Autodesk Inventor part; units mm, degrees
ref_plane "YZ Plane" through (0, 0, 0) normal (1, 0, 0) x (0, 1, 0)
ref_plane "XZ Plane" through (0, 0, 0) normal (0, 1, 0) x (-1, 0, 0)
ref_plane "XY Plane" through (0, 0, 0) normal (0, 0, 1) x (1, 0, 0)
sketch "Sketch1" plane through (0, 0, 0) normal (1, 0, 0) x (0, 1, 0)
  line L0 (-11.2229, 4.9257) -> (471.3771, 4.9257)
  line L1 (471.3771, 4.9257) -> (471.3771, -7.7743)
  line L2 (471.3771, -7.7743) -> (-11.2229, -7.7743)
  line L3 (-11.2229, -7.7743) -> (-11.2229, 4.9257)
  point P0 (0, 0)
  dimension "d0" = 482.6
revolve "Revolution1" add sketch "Sketch1" angle 360 about axis through (0, -11.2229, 4.9257) along (0, 1, 0)
sketch "Sketch2" plane through (0, 471.3771, 4.9257) normal (0, 1, 0) x (1, 0, 0)
  line L0 (-2.5588, -10.1161) -> (2.6183, -10.1161)
  line L1 (2.6183, -10.1161) -> (2.6183, 10.1161)
  line L2 (2.6183, 10.1161) -> (-2.5588, 10.1161)
  line L3 (-2.5588, 10.1161) -> (-2.5588, -10.1161)
  line L4 (-2.5588, 0) -> (2.6183, 0)
  point P0 (0, 4.9257)
extrude "Extrusion1" add sketch "Sketch2" along normal blind 95.25
sketch "Sketch3" plane through (2.6183, 471.3771, 15.0418) normal (1, 0, 0) x (0, 0, -1)
  line L0 (20.2322, 0) -> (0, 0)
  line L1 (20.2322, 0) -> (20.2322, 95.25)
  line L2 (0, 95.25) -> (20.2322, 95.25)
  line L3 (0, 0) -> (0, 95.25)
  line L4 (-2.5839, 0) -> (22.8161, 0)
  line L5 (10.1161, 0) -> (10.1161, 76.2)
  circle A0 centre (10.1161, 76.2) radius 12.7
  circle A1 centre (10.1161, 76.2) radius 19.05
  point P0 (15.0418, -471.3771)
  dimension "d10" = 76.2
  dimension "d11" = 25.4
  dimension "d12" = 38.1
extrude "Extrusion2" add sketch "Sketch3" against normal blind 6.35 contours A1 L5 A0 L1 | L1 A0 A1 | A1 L3 A0 L5 | A1 L3 A0 | A0 L3 A1 L1
sketch "Sketch4" plane through (2.6183, 471.3771, 15.0418) normal (1, 0, 0) x (0, 0, -1)
  line L0 (20.2322, 68.5218) -> (20.2322, 83.8782)
  arc A0 (20.2322, 68.5218) -> (20.2322, 83.8782) centre (10.1161, 76.2) ccw
  arc A1 (20.2322, 60.0579) -> (20.2322, 92.3421) centre (10.1161, 76.2) ccw
  line L1 (20.2322, 92.3421) -> (20.2322, 95.25)
  line L2 (0, 95.25) -> (20.2322, 95.25)
  line L3 (0, 92.3421) -> (0, 95.25)
  arc A2 (0, 92.3421) -> (0, 60.0579) centre (10.1161, 76.2) ccw
  line L4 (0, 0) -> (0, 60.0579)
  line L5 (20.2322, 0) -> (0, 0)
  line L6 (20.2322, 0) -> (20.2322, 60.0579)
  arc A3 (0, 83.8782) -> (0, 68.5218) centre (10.1161, 76.2) ccw
  line L7 (0, 68.5218) -> (0, 83.8782)
  arc A4 (0, 83.8782) -> (0, 68.5218) centre (10.1161, 76.2) ccw
  arc A5 (20.2322, 83.8782) -> (0, 83.8782) centre (10.1161, 76.2) ccw
  arc A6 (20.2322, 68.5218) -> (20.2322, 83.8782) centre (10.1161, 76.2) ccw
  arc A7 (0, 68.5218) -> (20.2322, 68.5218) centre (10.1161, 76.2) ccw
  circle A8 centre (10.1161, 76.2) radius 12.7
  point P0 (15.0418, -471.3771)
extrude "Extrusion3" cut sketch "Sketch4" against normal blind 6.35 contours A7 L7 A5 L0 | L0 A0 | A3 L7
properties part number "Rod"
For this review, take the finished solid that the model builds, in its own axes (mm). A direction names the side the tool comes from. Round coordinates to 2 decimals unless told otherwise and drop trailing zeros. Order: outer loops, then holes, each group sorted by start corner. A loop starts at its lowest first (then second) coordinate and runs counter-clockwise, first axis right, second up. Notation, with made-up numbers: M 55,-28.5 L 73,-28.5 A19 ccw 73,-16.5 Z; hole C -25.75,82.5 d10. An arc over 180 degrees is marked long. Use a Markdown table: item, result. Add a question column.
Item 1: Tool access review of faces 1 (the flat face through (-3.732, 535, 1)), 2 (the flat face through (0, -11.223, 5)), 3 (the flat face through (2.618, 518, 5)): name each direction out of +Z, -Z, +X, -X, +Y, -Y from which nothing blocks a thin tool from reaching the whole face with its end or side.
Item 2: Add section A-A, the plane y = 107.5. Give the boundary of the cut face in (x, z).
Item 3: Add section B-B, the plane x = 6.75. Give the boundary of the cut face in (y, z), then the cut area to 3 significant figures.
Item 4: To check wall thickness, follow line 1 along Y through (x, z) = (7.25, 5); line 2 along Z through (x, y) = (-1.5, 449); line 3 along X through (y, z) = (508, 12). State the ranges of each line that lie inside material, in increasing order.
Item 5: Insertion check: pin 1 (8 mm diameter, centred on x = 8.5, y = 502, fed in from -Z); pin 2 (2.5 mm diameter, centred on x = 0.5, y = 565, fed in from -Z); pin 3 (10 mm diameter, centred on y = 152, z = -5.5, fed in from +X); pin 4 (19 mm diameter, centred on y = 550, z = 12.5, fed in from -X). Each pin has a flat end and moves straight along its axis. Give the tip position at first contact, or say it passes through.
Geometry results:
| question | item | result |
|---|---|---|
| 1 | face 1 | +Z, -Z, -X, +Y |
| 1 | face 2 | +Z, -Z, +X, -X, -Y |
| 1 | face 3 | +Z, -Z, +X, +Y |
| 2 | outline | C 0,4.93 d25.4 |
| 3 | outline | M -11.22,-5.83 L 471.38,-5.83 L 471.38,15.68 L -11.22,15.68 Z |
| 3 | area | 10,400 mm² |
| 4 | line 1 | y = -11.22 to 471.38 |
| 4 | line 2 | z = -7.69 to 17.54 |
| 4 | line 3 | x = -2.56 to 2.62 |
| 5 | pin 1 | passes through |
| 5 | pin 2 | stops at z = -5.19 |
| 5 | pin 3 | stops at x = 11.48 |
| 5 | pin 4 | stops at x = -3.73 |
